from build123d import *

# Parameters (mm, degrees)
SKETCH1_W           = 114
SKETCH1_H           = 40
BOSS_EXTRUDE1_DEPTH = 3
CUT_EXTRUDE1_DEPTH  = 4
BOSS_EXTRUDE2_DEPTH = 3


with BuildPart() as part:
    # Sketch1 → Boss-Extrude1 (new body)
    with BuildSketch(Plane(origin=(0, 0, 0), x_dir=(1, 0, 0), z_dir=(0, 1, 0))):
        with Locations((-24.485507246, 12.735507246)):
            Rectangle(SKETCH1_W, SKETCH1_H)
    extrude(amount=BOSS_EXTRUDE1_DEPTH)

    # Sketch2 → Cut-Extrude1 (cut, through all)
    with BuildSketch(Plane(origin=(0, 3, 0), x_dir=(1, 0, 0), z_dir=(0, 1, 0))):
        Polygon((-36.485507246, 32.735507246), (-44.165937049, 25.055077444), (-47.560826058, 21.660188435), (-58.747394556, 21.660188435), (-72.532338505, 7.875244486), (-81.485507246, -1.077924256), (-81.485507246, 32.735507246), align=None)
    extrude(amount=-CUT_EXTRUDE1_DEPTH, mode=Mode.SUBTRACT)

    # Sketch3 → Boss-Extrude2 (add, through all)
    with BuildSketch(Plane(origin=(0, 3, 0), x_dir=(1, 0, 0), z_dir=(0, 1, 0))):
        Polygon((32.514492754, -7.264492754), (40.514492754, 0.735507246), (40.514492754, 32.735507246), (32.514492754, 32.735507246), align=None)
    extrude(amount=-BOSS_EXTRUDE2_DEPTH)


solid = part.part
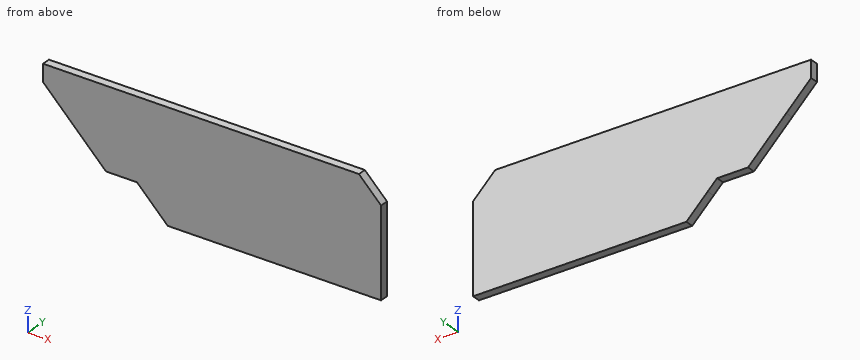
The model under review builds one solid part; all positions refer to its coordinate system, in mm. Round coordinates to 2 decimals unless told otherwise and drop trailing zeros. Loops run counter-clockwise (first coordinate to the right, second up) from the corner with the lowest first, then second, coordinate; pieces in that order, holes last. Notation, with made-up numbers: (53.5, -36.5) -> (60.5, -36.5) arc R32 ccw to (60.5, 0.5) -> close; hole circle Ø1 at (6.5, 30.5). An arc over 180 degrees is marked (long way). Return JSON: item names as keys, results as strings.
(1) For pin 1 (0.9 mm diameter, centred on x = -51, y = 1.5, fed in from -Z); pin 2 (1 mm diameter, centred on y = 2.5, z = -27.5, fed in from -X), all flat-tipped, find the tip position at first contact; note any pin that passes through.
Solved:
{"pin 1": "z = -21.66", "pin 2": "x = -42.22"}
(2) For line 1 (Z direction, x = -54, y = 2.55); line 2 (X direction, y = 0.95, z = -22.5); line 3 (X direction, y = 0.5, z = -5), list the stretches that pass through material, from the lowest coordinate up.
Solved:
{"line 1": "-21.66 to 7.26", "line 2": "-46.72 to 40.51", "line 3": "-75.41 to 40.51"}
(3) Add section A-A on y = 1.9. Write out the cut boundary in (x, z), plus the area to 3 significant figures.
Solved:
{"outline": "(-81.49, 1.08) -> (-58.75, -21.66) -> (-47.56, -21.66) -> (-36.49, -32.74) -> (40.51, -32.74) -> (40.51, -0.74) -> (32.51, 7.26) -> (-81.49, 7.26) -> close", "area": "4,150 mm2"}
(4) Add section B-B on z = -29. Write out the cut boundary in (x, y), plus the area to 3 significant figures.
Solved:
{"outline": "(-40.22, 0) -> (40.51, 0) -> (40.51, 3) -> (-40.22, 3) -> close", "area": "242 mm2"}
(5) Add section C-C on x = -64. Write out the cut boundary in (y, z).
Solved:
{"outline": "(0, -16.41) -> (3, -16.41) -> (3, 7.26) -> (0, 7.26) -> close"}
